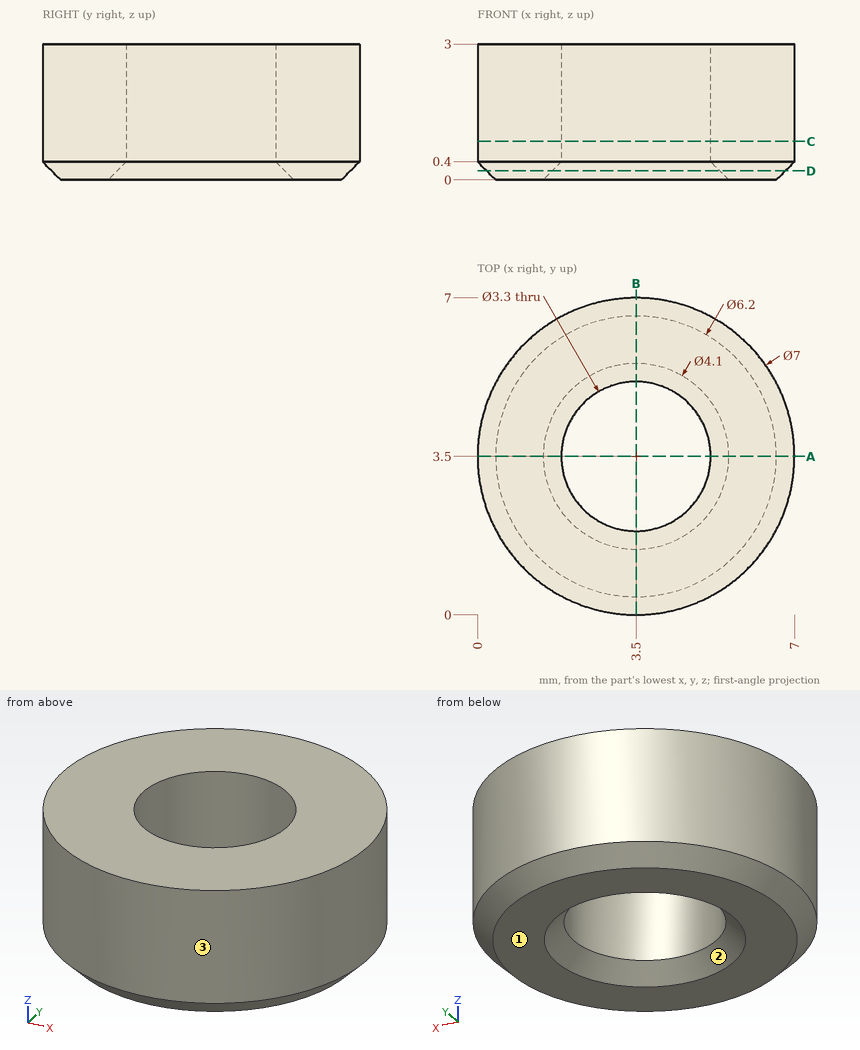
Source: three-view drawing plus pictorial views. Frame: mm from the lowest corner of the part. Give positions to 0.01 mm unless a question says otherwise; leave off trailing zeros. Order: outer loops, then holes, each group sorted by start corner. A loop starts at its lowest first (then second) coordinate and runs counter-clockwise, first axis right, second up. Notation, with made-up numbers: M -12.5,-10.5 L -4.5,-10.5 A22 cw -4.5,0.5 Z; hole C 31.5,30 d8. An arc over 180 degrees is marked long. Return JSON: item names as keys, results as strings.
Item 1: First-contact query: P1, Ø2, axis at x = 3.5, y = 3.5, coming from the +Z side. Flat tip, straight axial feed; report the tip coordinate or a pass-through.
Solutions:
{"P1": "through"}
Item 2: Ray query, probe 1 along Y at (x, z) = (3.5, 2.5); probe 2 along X at (y, z) = (2, 2.3); probe 3 along X at (y, z) = (3.25, 1.7). Return the intervals inside material, ascending.
Solutions:
{"probe 1": "0 to 1.85, 5.15 to 7", "probe 2": "0.34 to 2.81, 4.19 to 6.66", "probe 3": "0.01 to 1.87, 5.13 to 6.99"}
Item 3: Cut plane C-C (z = 0.85). Return loops of the section in (x, y), then the cut area to 3 significant figures.
Solutions:
{"outline": "C 3.5,3.5 d7; hole C 3.5,3.5 d3.3", "area": "29.9 mm^2"}
Item 4: Cut plane A-A (y = 3.5). Return loops of the section in (x, z), then the cut area to 3 significant figures.
Solutions:
{"outline": "M 0,0.4 L 0.4,0 L 1.45,0 L 1.85,0.4 L 1.85,3 L 0,3 Z; M 5.15,0.4 L 5.55,0 L 6.6,0 L 7,0.4 L 7,3 L 5.15,3 Z", "area": "10.8 mm^2"}
Item 5: Pull-direction query (Y, two-part tool) for the marked faces 1, 2 and 3; classes: +Y half, -Y half, draft (parallel to the pull), parting line (faces both ways), or undercut.
Solutions:
{"face 1": "draft", "face 2": "undercut", "face 3": "parting line"}
Item 6: Cut plane D-D (z = 0.2). Return loops of the section in (x, y).
Solutions:
{"outline": "C 3.5,3.5 d6.6; hole C 3.5,3.5 d3.7"}
